Design review of the part built by this model. Coordinates are the model's own, in mm. Face numbers are marked on the shaded views. Round coordinates to 2 decimals unless told otherwise and drop trailing zeros. Order: outer loops, then holes, each group sorted by start corner. A loop starts at its lowest first (then second) coordinate and runs counter-clockwise, first axis right, second up. Notation, with made-up numbers: M 26,26 L 78,26 A30 cw 78,63 Z; hole C 26.5,44 d5. An arc over 180 degrees is marked long. Use a Markdown table: item, result. Add a question column.
(1) The part is to be moulded in two halves that separate along X. For the marked faces 1, 2 and 3, say which applies: released by +X, released by -X, zero draft, split by the parting line, or undercut.
(2) To check wall thickness, follow probe 1 along Z at (x, y) = (0, -23.6) (3 decimals); probe 2 along Z at (x, y) = (0, -14.5) (3 decimals); probe 3 along Y at (x, z) = (14, -18.5). State the ranges of each line that lie inside material, in increasing order. Write a range as from..to.
(3) Take a section at B-B (y = -16). Write out the cut boundary in (x, z) (3 decimals), then the cut area to 3 significant figures.
(4) Take a section at C-C (x = 11). Write out the cut boundary in (y, z).
(5) For pin 1 (10 mm diameter, centred on y = -6.5, z = 8, fed in from +X); pin 2 (3 mm diameter, centred on y = -10, z = 2.5, fed in from +X); pin 3 (3 mm diameter, centred on x = 6.5, y = -19, fed in from -Z), all flat-tipped, find the tip position at first contact; note any pin that passes through.
(6) Take a section at A-A (x = -14.5). Write out the cut boundary in (y, z), then the cut area to 3 significant figures.
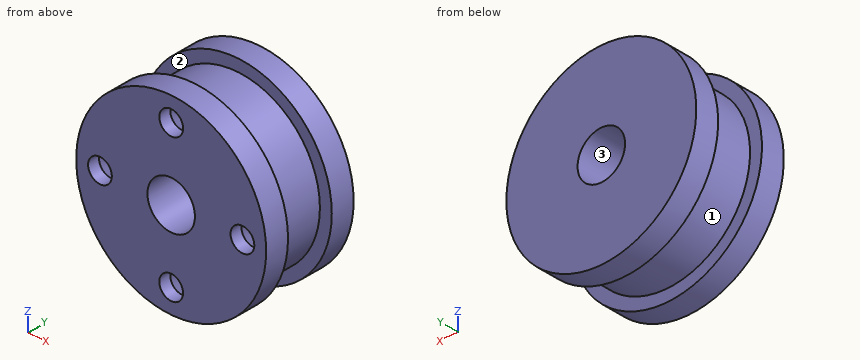
```python
from build123d import *

# Parameters (mm, degrees)
F0_R     = 25.4
F1_DEPTH = 6.35
F2_R     = 22.225
F3_DEPTH = 12.7
F4_R     = 25.4
F5_DEPTH = 6.35
F7_D     = 6.35
F7_DEPTH = 3.175
F7_TIP   = 1.9077324654
F9_D     = 12.7


with BuildPart() as f1:
    # F0 (on Front) → F1 (new body)
    with BuildSketch(Plane.XZ):
        Circle(F0_R)
    extrude(amount=F1_DEPTH)

    # F2 (on face) → F3 (join)
    with BuildSketch(Plane.XZ.offset(6.35)):
        Circle(F2_R)
    extrude(amount=F3_DEPTH)

    # F4 (on face) → F5 (join)
    with BuildSketch(Plane.XZ.offset(19.05)):
        Circle(F4_R)
    extrude(amount=F5_DEPTH)

    # F7
    with Locations(Plane.XZ.offset(25.4)):
        with Locations((-19.05, 0), (0, -19.05), (19.05, 0), (0, 19.05)):
            Hole(F7_D / 2, depth=F7_DEPTH)
            with Locations((0, 0, -(F7_DEPTH + F7_TIP / 2))):  # 118° drill point
                Cone(0, F7_D / 2, F7_TIP, mode=Mode.SUBTRACT)

    # F9 (through all)
    with Locations(Plane.XZ.offset(25.4)):
        with Locations((0, 0)):
            Hole(F9_D / 2)


solid = f1.part
```
Verdict:
| question | item | result |
|---|---|---|
| 1 | face 1 | split by the parting line |
| 1 | face 2 | zero draft |
| 1 | face 3 | undercut |
| 2 | probe 1 | z = -25.4..-22.225, -15.875..-6.35, 6.35..15.875, 22.225..25.4 |
| 2 | probe 2 | z = -22.225..-6.35, 6.35..22.225 |
| 2 | probe 3 | y = -25.4..-19.05, -6.35..0 |
| 3 | outline | C 0,0 d44.45; hole C 0,0 d12.7 |
| 3 | area | 1,430 mm^2 |
| 4 | outline | M -25.4,-22.89 L -19.05,-22.89 L -19.05,-19.31 L -6.35,-19.31 L -6.35,-22.89 L 0,-22.89 L 0,22.89 L -6.35,22.89 L -6.35,19.31 L -19.05,19.31 L -19.05,22.89 L -25.4,22.89 Z |
| 5 | pin 1 | stops at x = 25.22 |
| 5 | pin 2 | stops at x = 22.2 |
| 5 | pin 3 | stops at z = -24.9 |
| 6 | outline | M -25.4,-20.85 L -19.05,-20.85 L -19.05,-16.84 L -6.35,-16.84 L -6.35,-20.85 L 0,-20.85 L 0,20.85 L -6.35,20.85 L -6.35,16.84 L -19.05,16.84 L -19.05,20.85 L -25.4,20.85 Z |
| 6 | area | 958 mm^2 |
